Geometry check sheet. Reference: drawing and pictorial views, mm from the part's lowest x, y, z. Round coordinates to 2 decimals unless told otherwise and drop trailing zeros. Order: outer loops, then holes, each group sorted by start corner. A loop starts at its lowest first (then second) coordinate and runs counter-clockwise, first axis right, second up.
(1) Draft check along Z on the marked faces 1, 2, 3 and 4. Enter one of: pulls with the +Z half, pulls with the -Z half, needs draft (parallel to the pull), parting line crosses it, or undercut.
(2) Thickness scan on L1, parallel to Y at x = 12.5, z = 17.75 (1 decimal); L2, parallel to Y at x = 17, z = 8.25 (1 decimal); L3, parallel to Z at x = 33, y = 61.5. Record the ranges inside material, lowest first.
(3) Cross-section at B-B on y = 40. Enter the section's corners in (x, z).
(4) Cross-section at A-A on x = 17. Count the separate pieces of the cut face and the enclosed holes in it, and give its area (3 significant figures).
(5) Gauge pin test, flat ends, axial feed: P1, Ø2, axis at x = 20.5, z = 8.5, coming from the +Y side; P2, Ø12, axis at x = 12, z = 21.5, coming from the -Y side. Record the tip position at first contact, or that the pin passes through.
(6) Cross-section at C-C on z = 8.75. Enter the section's corners in (x, y), and give its area (3 significant figures).
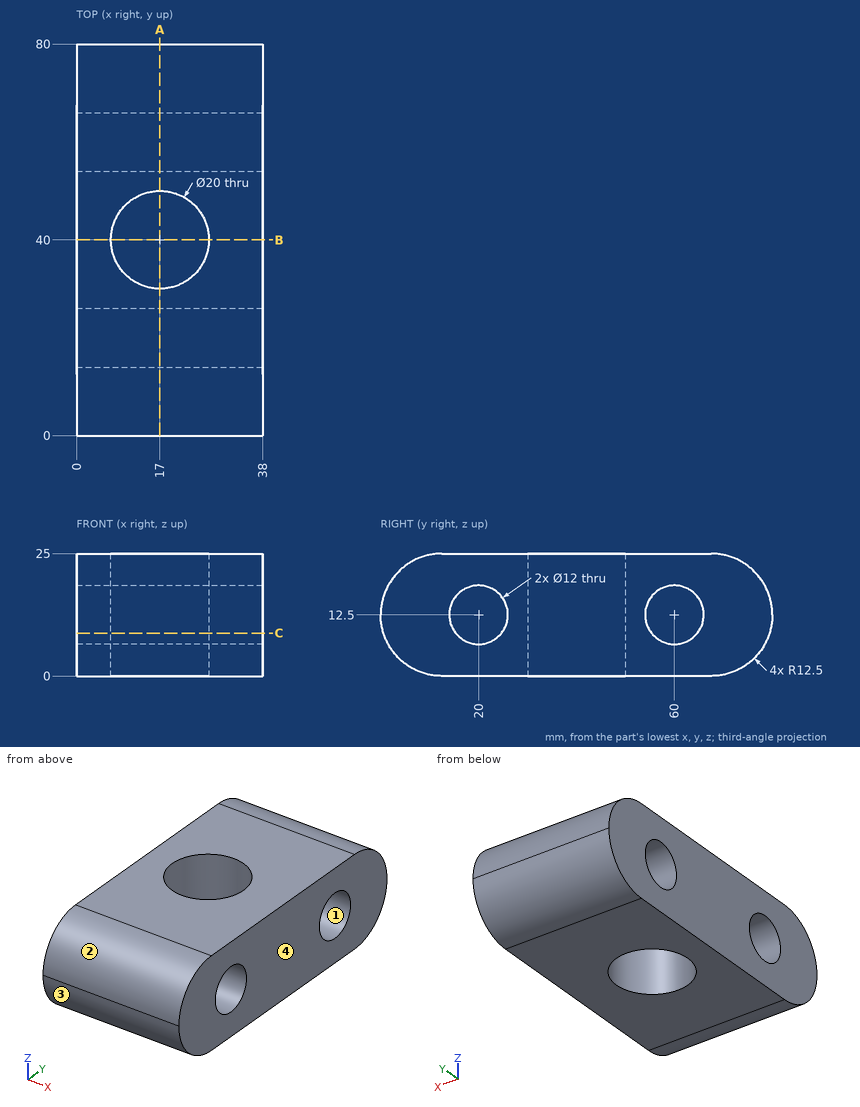
Found:
1. face 1: undercut
1. face 2: pulls with the +Z half
1. face 3: pulls with the -Z half
1. face 4: needs draft
2. L1: y = 1.2 to 17.1, 22.9 to 31.1, 48.9 to 57.1, 62.9 to 78.8
2. L2: y = 0.7 to 15.8, 24.2 to 30, 50 to 55.8, 64.2 to 79.3
2. L3: z = 0 to 6.69, 18.31 to 25
3. outline: (0, 0) - (7, 0) - (7, 25) - (0, 25) - close; (27, 0) - (38, 0) - (38, 25) - (27, 25) - close
4. separate pieces: 2
4. enclosed holes: 2
4. area: 1,140 mm2
5. P1: stops at y = 79.63
5. P2: stops at y = 0.37
6. outline: (0, 0.58) - (38, 0.58) - (38, 15.32) - (0, 15.32) - close; (0, 24.68) - (38, 24.68) - (38, 55.32) - (0, 55.32) - close; (0, 64.68) - (38, 64.68) - (38, 79.42) - (0, 79.42) - close; hole circle Ø20 at (17, 40)
6. area: 1,970 mm2
